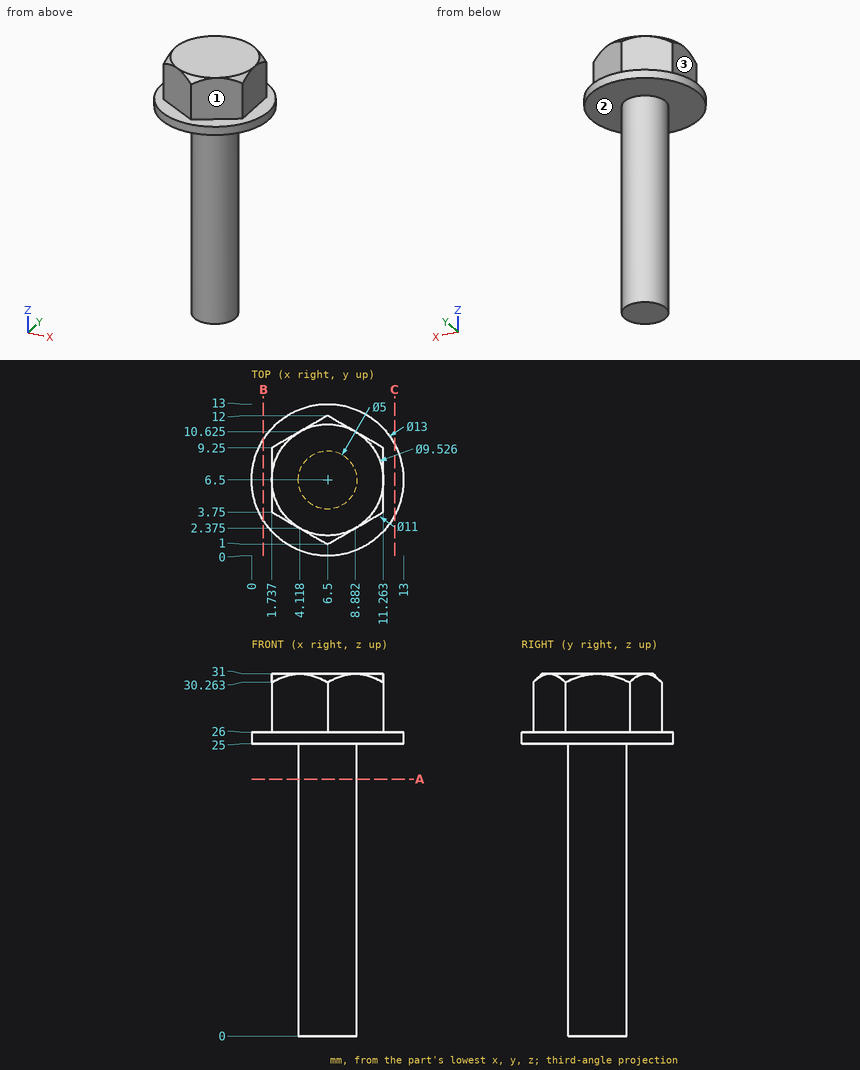
Could you check a few things on this drawing? It's one solid part, dimensions in mm from its lowest x, y, z. A direction names the side the tool comes from. Give positions to 0.01 mm unless a question says otherwise; leave off trailing zeros. Loops run counter-clockwise (first coordinate to the right, second up) from the corner with the lowest first, then second, coordinate; pieces in that order, holes last. Notation, with made-up numbers: (-0.75, -16) -> (38.25, -16) arc R26 cw to (38.25, -1) -> close; hole circle Ø3 at (23.5, 45.25). An arc over 180 degrees is marked (long way). Use one line per item in the form item = value. Start each with the question number.
1) Imagine slicing it at B-B (x = 1). Please give me the cut outline in (y, z) (1 decimal).
2) Imagine slicing it at C-C (x = 12.25). Please give me the cut outline in (y, z).
3) Which directions (+Z, -Z, +X, -X, +Y, -Y) give clear straight access to the entire face, cutting with the end or side of a thin tool? Please do the marked faces 1, 2 and 3.
4) Imagine slicing it at A-A (z = 22). Please give me the cut outline in (x, y).
5) Please list where these lines run through material, in increasing order: line 1 along Z through (x, y) = (9, 10.75); line 2 along Z through (x, y) = (11, 7); line 3 along X through (y, z) = (7.25, 12.5) (1 decimal).
6) For P1, Ø5, axis at x = 3.5, z = 8, coming from the +Y side; P2, Ø1, axis at x = 4.5, y = 11.5, coming from the +Z side; P3, Ø5, axis at y = 6.5, z = 7.5, coming from the -X side, each with a flat end and sliding along its axis, tell me the tip position at first contact or that it passes through.
Check values:
q1.outline = (3, 25) -> (10, 25) -> (10, 26) -> (3, 26) -> close
q2.outline = (3.47, 25) -> (9.53, 25) -> (9.53, 26) -> (3.47, 26) -> close
q3.face_1 = +Z, +X, -Y
q3.face_2 = -Z
q3.face_3 = +Z, -X, +Y, -Y
q4.outline = circle Ø5 at (6.5, 6.5)
q5.line_1 = 25 to 26
q5.line_2 = 25 to 31
q5.line_3 = 4.1 to 8.9
q6.P1 = 8.95
q6.P2 = 26
q6.P3 = 4
